The listing builds one solid part. Answer for the finished solid, in the listing's coordinates (mm). A direction names the side the tool comes from. Coordinates: 2 decimals unless noted, no trailing zeros. Write each loop counter-clockwise with the first axis right and the second up, starting at its lowest first coordinate (ties: lowest second). Pieces come first, ordered by that corner, then holes.
from build123d import *

# Parameters (mm, degrees)
SZKIC1_W                    = 12
SZKIC1_H                    = 5
DODANIE_WYCI_GNI_CIE1_DEPTH = 8.55
SZKIC2_R                    = 1.1
WYTNIJ_WYCI_GNI_CIE1_DEPTH  = 9.55
SZKIC3_W                    = 12
SZKIC3_H                    = 2
WYTNIJ_WYCI_GNI_CIE2_DEPTH  = 1


with BuildPart() as part:
    # Szkic1 → Dodanie-wyciągnięcie1 (new body)
    with BuildSketch(Plane.XY):
        Rectangle(SZKIC1_W, SZKIC1_H)
    extrude(amount=DODANIE_WYCI_GNI_CIE1_DEPTH)

    # Szkic2 → Wytnij-wyciągnięcie1 (cut, through all)
    with BuildSketch(Plane.XY.offset(8.55)):
        with Locations((0, -0.15)):
            Circle(SZKIC2_R)
    extrude(amount=-WYTNIJ_WYCI_GNI_CIE1_DEPTH, mode=Mode.SUBTRACT)

    # Szkic3 → Wytnij-wyciągnięcie2 (cut)
    with BuildSketch(Plane(origin=(0, -2.5, 0), x_dir=(-1, 0, 0), z_dir=(0, -1, 0))):
        with Locations((0, -4.55)):
            Rectangle(SZKIC3_W, SZKIC3_H)
    extrude(amount=-WYTNIJ_WYCI_GNI_CIE2_DEPTH, mode=Mode.SUBTRACT)


solid = part.part
1. Find the intervals of material crossed by L1, parallel to Y at x = 0, z = 6.5; L2, parallel to Z at x = 0, y = -2; L3, parallel to Y at x = 0, z = 4, in increasing order.
Results found:
L1: y = -2.5 to -1.25, 0.95 to 2.5
L2: z = 0 to 3.55, 5.55 to 8.55
L3: y = -1.5 to -1.25, 0.95 to 2.5
2. A tool of negligible diameter and unlimited length cuts with its end or side. For faces 4 (the flat face through (0, -2.5, 7)), 5 (the flat face through (0, -1.5, 5)), from which of +Z, -Z, +X, -X, +Y, -Y can it reach the whole face along a straight path? Write none if from no direction.
Results found:
face 4: +Z, -Z, +X, -X, -Y
face 5: +X, -X, -Y
3. Section B-B on y = -0.15 is taken. Give the vertices of the cut face in (x, z).
Results found:
outline: (-6, 0) - (-1.1, 0) - (-1.1, 8.55) - (-6, 8.55) - close; (1.1, 0) - (6, 0) - (6, 8.55) - (1.1, 8.55) - close
4. Section D-D on x = 3.5 is taken. Give the vertices of the cut face in (y, z), then the cut area to 4 significant figures.
Results found:
outline: (-2.5, 0) - (2.5, 0) - (2.5, 8.55) - (-2.5, 8.55) - (-2.5, 5.55) - (-1.5, 5.55) - (-1.5, 3.55) - (-2.5, 3.55) - close
area: 40.75 mm2
5. For a pull along Z with two mould halves and no side action, classify faces 1 (the flat face through (-0.1, 1.1, 8.55)), 2 (the flat face through (0, -2, 3.55)), 3 (the flat face through (0, 2.5, 4)) as pulls with the +Z half, pulls with the -Z half, needs draft (parallel to the pull), parting line crosses it, or undercut.
Results found:
face 1: pulls with the +Z half
face 2: undercut
face 3: needs draft
6. Section C-C on z = 2 is taken. Give the vertices of the cut face in (x, y), then the cut area to 3 significant figures.
Results found:
outline: (-6, -2.5) - (6, -2.5) - (6, 2.5) - (-6, 2.5) - close; hole circle Ø2.2 at (0, -0.15)
area: 56.2 mm2
7. Section A-A on x = 0 is taken. Give the vertices of the cut face in (y, z), then the cut area to 3 significant figures.
Results found:
outline: (-2.5, 0) - (-1.25, 0) - (-1.25, 8.55) - (-2.5, 8.55) - (-2.5, 5.55) - (-1.5, 5.55) - (-1.5, 3.55) - (-2.5, 3.55) - close; (0.95, 0) - (2.5, 0) - (2.5, 8.55) - (0.95, 8.55) - close
area: 21.9 mm2
8. A flat-ended cylindrical pin translates along its axis: P1, Ø0.6, axis at x = 0, z = 4.5, coming from the -Y side. Find the tip coordinate at first contact, or state that the pin passes through.
Results found:
P1: stops at y = -1.5
